Design review of the part built by this model. Coordinates are the model's own, in mm. Face numbers are marked on the shaded views. A direction names the side the tool comes from. Give positions to 0.01 mm unless a question says otherwise; leave off trailing zeros. Write each loop counter-clockwise with the first axis right and the second up, starting at its lowest first coordinate (ties: lowest second). Pieces come first, ordered by that corner, then holes. Notation, with made-up numbers: M 1,-33 L 23,-33 A33 ccw 23,0 Z; hole C -40,11.25 d10. An arc over 180 degrees is marked long. Answer in a Markdown table with one row per item.
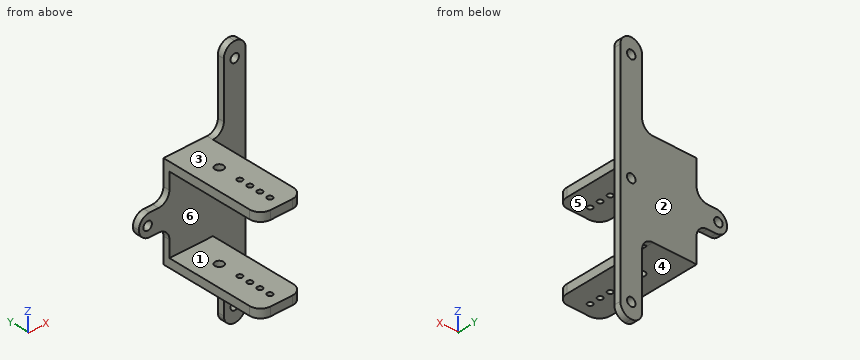
Autodesk Inventor part; units mm, degrees
ref_plane "YZ Plane" through (0, 0, 0) normal (1, 0, 0) x (0, 1, 0)
ref_plane "XZ Plane" through (0, 0, 0) normal (0, 1, 0) x (-1, 0, 0)
ref_plane "XY Plane" through (0, 0, 0) normal (0, 0, 1) x (1, 0, 0)
sketch "Szkic1" plane through (0, 0, 0) normal (0, 1, 0) x (-1, 0, 0)
  line L0 (9, 129.5) -> (-1, 129.5)
  line L1 (-1, 129.5) -> (-1, 15.5)
  line L2 (-1, 15.5) -> (9, 15.5)
  line L3 (9, 15.5) -> (9, 129.5)
  circle A0 centre (4, 22.5) radius 1.95
  circle A1 centre (4, 122.5) radius 1.95
  line L4 (48, 148) -> (48, 0)
  line L5 (9, 77.5) -> (48, 77.5)
  line L6 (48, 77.5) -> (48, 67.5)
  line L7 (48, 67.5) -> (9, 67.5)
  line L8 (9, 67.5) -> (9, 77.5)
  circle A2 centre (44, 72.5) radius 1.95
  line L9 (34, 94) -> (9, 94)
  line L10 (9, 94) -> (9, 51)
  line L11 (9, 51) -> (34, 51)
  line L12 (34, 51) -> (34, 94)
  circle A3 centre (4, 72.5) radius 1.95
  line L13 (34, 90) -> (9, 90) construction
  line L14 (9, 90) -> (9, 55) construction
  line L15 (9, 55) -> (34, 55) construction
  line L16 (34, 55) -> (34, 90) construction
  line L17 (34, 94) -> (14, 94)
  line L18 (14, 94) -> (14, 90)
  line L19 (14, 90) -> (34, 90)
  line L20 (34, 90) -> (34, 94)
  line L21 (14, 51) -> (34, 51)
  line L22 (34, 51) -> (34, 55)
  line L23 (34, 55) -> (14, 55)
  line L24 (14, 55) -> (14, 51)
  circle A4 centre (24, 47.5) radius 1.95
  circle A5 centre (24, 97.5) radius 1.95
  point P0 (0, 0)
  point P1 (12.3183, 7)
  dimension "d0" = 7
  dimension "d1" = 7
  dimension "d2" = 5
  dimension "d3" = 5
  dimension "d4" = 5
  dimension "d5" = 5
  dimension "d6" = 43
  dimension "d7" = 16.5
  dimension "d8" = 25
  dimension "d9" = 35
  dimension "d10" = 12.5
  dimension "d11" = 10
extrude "Wyciągnięcie proste1" add sketch "Szkic1" along normal blind 3 contours L3 L2 L1 L0 | L9 L18 L19 L12 L5 L3 | L5 L12 L7 L3 | L9 L12 L19 L18 | L7 L12 L23 L24 L11 L3 | L5 L4 L7 L12 | L24 L23 L12 L11
extrude "Wyciągnięcie proste2" add sketch "Szkic1" against normal blind 45 contours L9 L12 L19 L18 | L24 L23 L12 L11
fillet "Zaokrąglenie1" radius 5 14 edges at (-34, 1.5, 67.5) (-34, 1.5, 77.5) (-48, 1.5, 77.5) (-48, 1.5, 67.5) (-9, 1.5, 51) (-9, 1.5, 15.5) (1, 1.5, 15.5) (-9, 1.5, 94) (-9, 1.5, 129.5) (1, 1.5, 129.5) (-34, -45, 92) (-34, -45, 53) (-14, -45, 53) (-14, -45, 92)
sketch "Szkic2" plane through (-14, 3, 51) normal (0, 0, -1) x (-1, 0, 0)
  arc A0 (0, -43) -> (5, -48) centre (5, -43) ccw
  line L0 (15, -48) -> (5, -48)
  arc A1 (15, -48) -> (20, -43) centre (15, -43) ccw
  line L1 (20, -43) -> (20, 0)
  line L2 (0, 0) -> (20, 0)
  line L3 (0, -3) -> (0, 0)
  line L4 (0, -3) -> (0, -43)
  line L5 (-5, -3) -> (20, -3)
  point P0 (-14, -3)
  point P1 (10, -17)
  point P2 (10, -27.25)
  point P3 (10, -32.25)
  point P4 (10, -37.25)
  point P5 (10, -42.25)
  dimension "d17" = 14
  dimension "d18" = 10
  dimension "d19" = 10.25
  dimension "d20" = 5
  dimension "d21" = 5
  dimension "d22" = 5
hole "Otwór1" at (-24, -24.25, 51) at (-24, -29.25, 51) at (-24, -34.25, 51) at (-24, -39.25, 51) direction (0, 0, 1) diameter 2.4 end through all
hole "Otwór2" at (-24, -14, 51) direction (0, 0, 1) diameter 3.9 end through all
equation "\"d3\" = d2"
equation "\"d5\" = d4"
properties part number "czesc_do_obudowy"
1) Add section C-C (y = -18). Write out the cut boundary in (x, z), and give its area (3 significant figures).
Geometry says:
| item | result |
|---|---|
| outline | M -34,51 L -14,51 L -14,55 L -34,55 Z; M -34,90 L -14,90 L -14,94 L -34,94 Z |
| area | 160 mm^2 |
2) To check wall thickness, follow probe 1 along Z at (x, y) = (-4, 1.1); probe 2 along Y at (x, z) = (-24, 52.9); probe 3 along X at (y, z) = (-39.25, 91.9). State the ranges of each line that lie inside material, in increasing order. Write a range as [from, to].
Geometry says:
| item | result |
|---|---|
| probe 1 | [15.5, 20.55], [24.45, 70.55], [74.45, 120.55], [124.45, 129.5] |
| probe 2 | [-45, -40.45], [-38.05, -35.45], [-33.05, -30.45], [-28.05, -25.45], [-23.05, -15.95], [-12.05, 3] |
| probe 3 | [-34, -25.2], [-22.8, -14] |
3) Insertion check: P1, Ø6, axis at x = -44, z = 72.5, coming from the -Y side; P2, Ø3, axis at x = -11.5, z = 103, coming from the -Y side; P3, Ø1.5, axis at x = -41, y = 1.5, coming from the -Z side; P4, Ø3.5, axis at y = 2, z = 118, coming from the -X side. Each pin has a flat end and moves straight along its axis. Give the tip position at first contact, or say it passes through.
Geometry says:
| item | result |
|---|---|
| P1 | y = 0 |
| P2 | through |
| P3 | z = 67.5 |
| P4 | x = -9 |
4) Add section D-D (x = -24). Count the separate pieces of the cut face and the enclosed holes in it, and give its area (3 significant figures).
Geometry says:
| item | result |
|---|---|
| separate pieces | 11 |
| enclosed holes | 0 |
| area | 381 mm^2 |
5) The part is to be moulded in two halves that separate along Z. For the marked faces 3, 4, 5 and 6, say which applies: released by +Z, released by -Z, zero draft, split by the parting line, or undercut.
Geometry says:
| item | result |
|---|---|
| face 3 | released by +Z |
| face 4 | released by -Z |
| face 5 | undercut |
| face 6 | undercut |
6) Add section A-A (z = 22.5). Write out the cut boundary in (x, y), and give its area (3 significant figures).
Geometry says:
| item | result |
|---|---|
| outline | M -9,0 L -5.95,0 L -5.95,3 L -9,3 Z; M -2.05,0 L 1,0 L 1,3 L -2.05,3 Z |
| area | 18.3 mm^2 |
7) Add section B-B (y = -24.25). Write out the cut boundary in (x, z).
Geometry says:
| item | result |
|---|---|
| outline | M -34,51 L -25.2,51 L -25.2,55 L -34,55 Z; M -34,90 L -25.2,90 L -25.2,94 L -34,94 Z; M -22.8,51 L -14,51 L -14,55 L -22.8,55 Z; M -22.8,90 L -14,90 L -14,94 L -22.8,94 Z |
8) For the marked faces 1 and 2, list the 3-axis set-ups (+Z, -Z, +X, -X, +Y, -Y) from which the entire face can be reached by the end or side of a thin tool; tool diameter is ignored.
Geometry says:
| item | result |
|---|---|
| face 1 | +X, -X, -Y |
| face 2 | +Z, -Z, +X, -X, +Y |
